Answer from the drawing. Dimensions are ordinates in mm from the lowest x, y and z of the part. Coordinates: 2 decimals unless noted, no trailing zeros. Write each loop counter-clockwise with the first axis right and the second up, starting at its lowest first coordinate (ties: lowest second). Pieces come first, ordered by that corner, then holes. Notation, with made-up numbers: M -6,34 L 2,34 A16 ccw 2,52 Z; hole C 82,-36.75 d7. An arc over 180 degrees is marked long. Put each result on its own line as item: value. Start each with the question number.
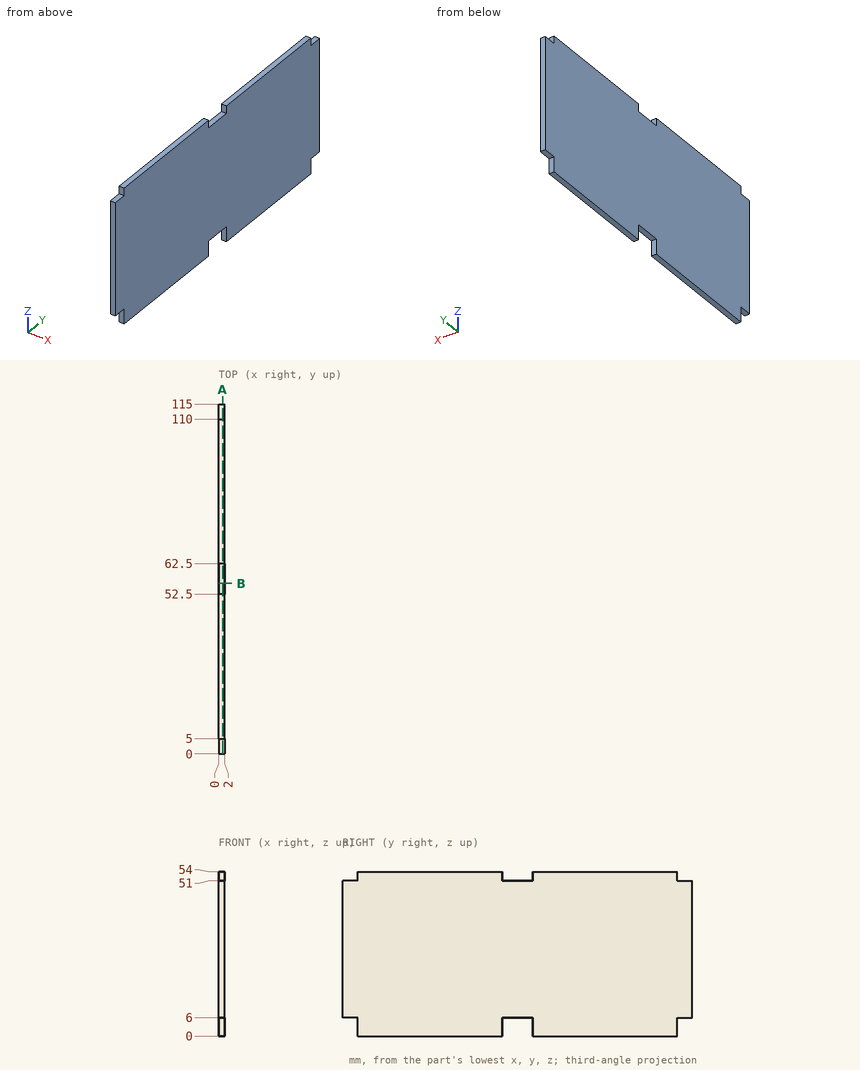
1) A cutting plane is placed at B-B on y = 56. Write down the section's boundary in (x, z), then the cut area to 3 significant figures.
2) Straight lines are drawn through the part: probe 1 along Y at (x, z) = (1.05, 5); probe 2 along Z at (x, y) = (0.65, 57). For each, find the intervals that lie inside material, in ascending order.
3) Given pin 1 Ø1 at (x, z) = (1, 2) entering from +Y; pin 2 Ø0.6 at (x, z) = (1, 3) entering from -Y; pin 3 Ø0.6 at (x, y) = (1, 111.5) entering from +Z, each flat-ended and moving along its own axis, determine where each tip first touches the part or whether it passes through.
4) A cutting plane is placed at A-A on x = 1.35. Write down the section's boundary in (y, z).
Answers follow:
1. outline: M 0,6 L 2,6 L 2,51 L 0,51 Z
1. area: 90.0 mm²
2. probe 1: y = 5 to 52.5, 62.5 to 110
2. probe 2: z = 6 to 51
3. pin 1: stops at y = 110
3. pin 2: stops at y = 5
3. pin 3: stops at z = 51
4. outline: M 0,6 L 5,6 L 5,0 L 52.5,0 L 52.5,6 L 62.5,6 L 62.5,0 L 110,0 L 110,6 L 115,6 L 115,51 L 110,51 L 110,54 L 62.5,54 L 62.5,51 L 52.5,51 L 52.5,54 L 5,54 L 5,51 L 0,51 Z
